Build history of the part. All positions in model axes, mm. A direction names the side the tool comes from. Give positions to 0.01 mm unless a question says otherwise; leave off trailing zeros. Order: outer loops, then holes, each group sorted by start corner. A loop starts at its lowest first (then second) coordinate and runs counter-clockwise, first axis right, second up. Notation, with made-up numbers: (18, 59) - (71, 59) arc R36 cw to (71, 97) - close; hole circle Ø6 at (55, 65). An arc over 180 degrees is marked (long way). Use a Markdown table: item, result. Add a question column.
(1) Slice it at C-C (z = -3). Write the cut outline in (x, y).
(2) Slice it at A-A (z = -7.75). Write the cut outline in (x, y), then the cut area to 3 significant figures.
(3) Slice it at B-B (y = 1.25). Write the cut outline in (x, z).
(4) Wall check: line 1 (Z direction, x = 0, y = 4.5); line 2 (Y direction, x = -4, z = 3.25); line 3 (Z direction, x = -5, y = 6). Give the ranges that are in metal, low to high.
(5) Flat gauge pins, fed straight in: pin 1 (1.5 mm diameter, centred on x = -7, y = 1, fed in from +Z); pin 2 (0.8 mm diameter, centred on x = 13, z = 1, fed in from +Y); pin 3 (1.7 mm diameter, centred on x = 13, y = 4, fed in from -Z). Where does each tip first touch, or does it go through?
(6) Mould opens along X. For faces 4 (the face through (-1.934, -1.014, 1.321)), 5 (the face through (2.5, 0, 0.2)), 6 (the face through (13, 2.5, 0)) say: +X half, -X half, draft (parallel to the pull), parting line (faces both ways), or undercut.
(7) Which spindle directions (+Z, -Z, +X, -X, +Y, -Y) get a long thin tool onto all of the face, cutting with end or side? Do faces 1 (the face through (1.1, 7, 12.4)), 2 (the face through (-5.537, 3.451, 10.646)), 3 (the face through (12, 5, -4)). Say none if no direction does.
Autodesk Inventor part; units mm, degrees
ref_plane "YZ Plane" through (0, 0, 0) normal (1, 0, 0) x (0, 1, 0)
ref_plane "XZ Plane" through (0, 0, 0) normal (0, 1, 0) x (-1, 0, 0)
ref_plane "XY Plane" through (0, 0, 0) normal (0, 0, 1) x (1, 0, 0)
sketch "Sketch1" plane through (0, 0, 0) normal (0, 1, 0) x (-1, 0, 0)
  circle A0 centre (0, 0) radius 14
  circle A1 centre (0, 0) radius 12
  dimension "d0" = 28
  dimension "d1" = 24
extrude "Extrusion1" add sketch "Sketch1" along normal blind 7
sketch "Sketch2" plane through (0, 7, 0) normal (0, 1, 0) x (1, 0, 0)
  line L0 (14, -4) -> (-14, -4)
  line L1 (-14, -4) -> (-14, 4)
  line L2 (-14, 4) -> (14, 4)
  line L3 (14, 4) -> (14, -4)
  line L4 (14, -4) -> (-14, 4) construction
  line L5 (-14, -4) -> (14, 4) construction
  line L6 (-0.5, 5) -> (0.5, 5)
  line L7 (0.5, 5) -> (0.5, -5)
  line L8 (0.5, -5) -> (-0.5, -5)
  line L9 (-0.5, -5) -> (-0.5, 5)
  line L10 (-0.5, 5) -> (0.5, -5) construction
  line L11 (0.5, 5) -> (-0.5, -5) construction
  point P0 (0, 0)
  dimension "d4" = 28
  dimension "d5" = 8
extrude "Extrusion2" cut sketch "Sketch2" against normal blind 8 contours L0 L7 L2 L3 | L0 L9 L2 L7 | L0 L1 L2 L9
sketch "Sketch3" plane through (0, 0, 0) normal (0, -1, 0) x (1, 0, 0)
  circle A0 centre (0, 0) radius 14
  dimension "d17" = 28
extrude "Extrusion3" add sketch "Sketch3" along normal blind 2
sketch "Sketch5" plane through (0, 0, 0) normal (0, 1, 0) x (1, 0, 0)
  point P0 (0, 0)
  point P1 (-0.0372, -0.1116)
hole "Hole2" at (-0.0372, 0, 0.1116) direction (0, -1, 0) diameter 4.5 end through all
extrude "Extrusion4" add sketch "Sketch1" along normal blind 2.5
properties part number "magneticslotV1"
Solution:
| question | item | result |
|---|---|---|
| 1 | outline | (-13.67, -2) - (13.67, -2) - (13.67, 2.5) - (11.62, 2.5) - (11.62, 0) - (-11.62, 0) - (-11.62, 2.5) - (-13.67, 2.5) - close |
| 2 | outline | (-11.66, -2) - (11.66, -2) - (11.66, 7) - (9.16, 7) - (9.16, 0) - (-9.16, 0) - (-9.16, 7) - (-11.66, 7) - close |
| 2 | area | 81.6 mm2 |
| 3 | outline | circle Ø28 at (0, 0); hole circle Ø24 at (0, 0) |
| 4 | line 1 | -14 to -12, 12 to 14 |
| 4 | line 2 | -2 to 0 |
| 4 | line 3 | -13.08 to -10.91, 10.91 to 13.08 |
| 5 | pin 1 | z = 12.53 |
| 5 | pin 2 | y = 2.5 |
| 5 | pin 3 | z = -6.96 |
| 6 | face 4 | undercut |
| 6 | face 5 | undercut |
| 6 | face 6 | draft |
| 7 | face 1 | +Z, -Z, +X, -X, +Y |
| 7 | face 2 | +Y |
| 7 | face 3 | +X, -X, +Y |
